Build history of the part. All positions in model axes, mm. A direction names the side the tool comes from. Give positions to 0.01 mm unless a question says otherwise; leave off trailing zeros. Write each loop counter-clockwise with the first axis right and the second up, starting at its lowest first coordinate (ties: lowest second). Pieces come first, ordered by that corner, then holes. Notation, with made-up numbers: M -32,57.5 L -23,57.5 A27 cw -23,78.5 Z; hole C -39,63 d6. An arc over 180 degrees is marked long. Return JSON: item names as keys, results as strings. Group by question number.
Q1. Tool access for faces 4 (the cylindrical face through (-1.2, -0.5, 11.6)), 5 (the flat face through (0, 5, 0)): list every direction of +Z, -Z, +X, -X, +Y, -Y with a clear straight run to the whole face (end or side of a thin tool).
Q2. Band-saw the part on A-A, the plane y = 7. Give the cut face in (x, z), then the cut area to 3 significant figures.
Q3. Pull direction X, two halves, no side cores. Call faces 1 (the conical face through (33.19, 12.85, 7.37)), 2 (the cylindrical face through (0.1, -0.83, 27.32)), 3 (the flat face through (0, -3, 0)): +X half, -X half, draft (parallel to the pull), parting line (faces both ways), or undercut.
Q4. Wall check: probe 1 along X at (y, z) = (-0.25, 0); probe 2 along Y at (x, z) = (-8, -7); probe 3 along Z at (x, y) = (-6, 59). Give the ranges that are in metal, low to high.
Q5. Flat gauge pins, fed straight in: pin 1 Ø2 at (x, z) = (-12, -3) entering from +Y; pin 2 Ø3.5 at (x, z) = (0, 10) entering from -Y; pin 3 Ø2 at (x, y) = (20.5, 49) entering from +Z; pin 4 Ø6 at (x, y) = (4, 27) entering from -Z. Where does each tip first touch, or does it go through?
from build123d import *

# Parameters (mm, degrees)
SKETCH4_R               = 33
SKETCH4_R_2             = 2
BOSS_EXTRUDE1_DEPTH     = 3
SKETCH8_R               = 36.5
SKETCH9_R               = 45
SKETCH8_3_R             = 35.5
SKETCH9_3_R             = 44
FILLET1_R               = 100
FILLET2_R               = 100
BOSS_EXTRUDE2_START     = 5
SKETCH10_R              = 27.5
SKETCH10_R_2            = 2
BOSS_EXTRUDE2_DEPTH     = 5
CUT_EXTRUDE1_DEPTH      = 95.604439811
CUT_EXTRUDE1_DEPTH_BACK = 95.604439811
SKETCH11_R              = 2.340885688
SKETCH12_R              = 4
CUT_EXTRUDE2_DEPTH      = 3


with BuildPart() as part:
    # Sketch2 → Revolve1 (revolve)
    with BuildSketch(Plane(origin=(0, 0, 0), x_dir=(0, 0, -1), z_dir=(1, 0, 0)), mode=Mode.PRIVATE) as revolve1_sk:
        Polygon((-32, 0), (-33, 0), (-36.5, 45), (-35.5, 45), align=None)
    revolve(revolve1_sk.sketch.rotate(Axis((0, 0, 0), (0, 1, 0)), 180), axis=Axis((0, 0, 0), (0, 1, 0)))

    # Sketch4 → Boss-Extrude1 (add)
    with BuildSketch(Plane.XZ):
        with Locations(Location((0, 0, 0), (0, 0, 270))):
            Circle(SKETCH4_R)
        with Locations(Location((0, 10, 0), (0, 0, 270))):
            Circle(SKETCH4_R_2, mode=Mode.SUBTRACT)
        with Locations(Location((0, -5, 0), (0, 0, 270))):
            Circle(SKETCH4_R_2, mode=Mode.SUBTRACT)
    extrude(amount=BOSS_EXTRUDE1_DEPTH)

    # Sketch8 → Loft1 section 0
    with BuildSketch(Plane(origin=(0, 45, 0), x_dir=(1, 0, 0), z_dir=(0, 1, 0))):
        Circle(SKETCH8_R)
    # Sketch9 → Loft1 section 1
    with BuildSketch(Plane(origin=(0, 70, 0), x_dir=(1, 0, 0), z_dir=(0, 1, 0))):
        Circle(SKETCH9_R)
    loft()

    # Sketch8<3> → Cut-Loft1 section 0
    with BuildSketch(Plane(origin=(0, 45, 0), x_dir=(1, 0, 0), z_dir=(0, 1, 0))):
        Circle(SKETCH8_3_R)
    # Sketch9<3> → Cut-Loft1 section 1
    with BuildSketch(Plane(origin=(0, 70, 0), x_dir=(1, 0, 0), z_dir=(0, 1, 0))):
        Circle(SKETCH9_3_R)
    loft(mode=Mode.SUBTRACT)

    # Fillet1
    fillet1_edges = [part.edges().sort_by_distance(p)[0] for p in [
        (-25.102290732, 45, 25.102290732),
    ]]
    fillet(fillet1_edges, radius=FILLET1_R)

    # Fillet2
    fillet2_edges = [part.edges().sort_by_distance(p)[0] for p in [
        (-25.809397513, 45, 25.809397513),
    ]]
    fillet(fillet2_edges, radius=FILLET2_R)

    # Sketch10 → Boss-Extrude2 (add)
    with BuildSketch(Plane(origin=(0, 0, 0), x_dir=(1, 0, 0), z_dir=(0, 1, 0)).offset(BOSS_EXTRUDE2_START)):
        with Locations(Location((0, 0, 0), (0, 0, 90))):
            Circle(SKETCH10_R)
        with Locations(Location((0, 5, 0), (0, 0, 90))):
            Circle(SKETCH10_R_2, mode=Mode.SUBTRACT)
        with Locations(Location((0, -10, 0), (0, 0, 90))):
            Circle(SKETCH10_R_2, mode=Mode.SUBTRACT)
    extrude(amount=-BOSS_EXTRUDE2_DEPTH)

    # Sketch11 → Cut-Extrude1 (cut, two sides: drawn at the far end of the back side and taken through both)
    with BuildSketch(Plane(origin=(0, 0, 0), x_dir=(1, 0, 0), z_dir=(0, 1, 0)).offset(-CUT_EXTRUDE1_DEPTH_BACK)):
        with Locations(Location((0, 29.659114312, 0), (0, 0, 270))):
            Circle(SKETCH11_R)
        with Locations(Location((29.659114312, 0, 0), (0, 0, 270))):
            Circle(SKETCH11_R)
        with Locations(Location((0, -29.659114312, 0), (0, 0, 270))):
            Circle(SKETCH11_R)
        with Locations(Location((-29.659114312, 0, 0), (0, 0, 270))):
            Circle(SKETCH11_R)
    extrude(amount=CUT_EXTRUDE1_DEPTH + CUT_EXTRUDE1_DEPTH_BACK, mode=Mode.SUBTRACT)

    # Sketch12 → Cut-Extrude2 (cut)
    with BuildSketch(Plane(origin=(0, 5, 0), x_dir=(1, 0, 0), z_dir=(0, 1, 0))):
        with Locations(Location((0, 5, 0), (0, 0, 270))):
            Circle(SKETCH12_R)
        with Locations(Location((0, -10, 0), (0, 0, 270))):
            Circle(SKETCH12_R)
    extrude(amount=-CUT_EXTRUDE2_DEPTH, mode=Mode.SUBTRACT)


solid = part.part
From the geometry:
{
 "1": {"face 4": "+Y, -Y", "face 5": "+Y"},
 "2": {"outline": "C 0,0 d67.09; hole C 0,0 d65.09", "area": "208 mm^2"},
 "3": {"face 1": "parting line", "face 2": "undercut", "face 3": "draft"},
 "4": {"probe 1": "x = -33 to -32, -27.32 to 27.32, 32 to 33", "probe 2": "y = -3 to 5", "probe 3": "z = -40.82 to -39.81, 39.81 to 40.82"},
 "5": {"pin 1": "stops at y = 5", "pin 2": "passes through", "pin 3": "stops at z = 32.94", "pin 4": "stops at z = -35.22"}
}
